For this review, take the finished solid that the model builds, in its own axes (mm). Face numbers are marked on the shaded views. Give positions to 0.01 mm unless a question says otherwise; leave off trailing zeros. Write each loop counter-clockwise with the first axis right and the second up, starting at its lowest first coordinate (ties: lowest second). Pieces come first, ordered by that corner, then holes. Notation, with made-up numbers: (-22, 46) -> (-9, 46) arc R35 cw to (-9, 84) -> close; hole circle Ø8 at (86.25, 2). An arc over 180 degrees is marked (long way). Return JSON: item names as keys, results as strings.
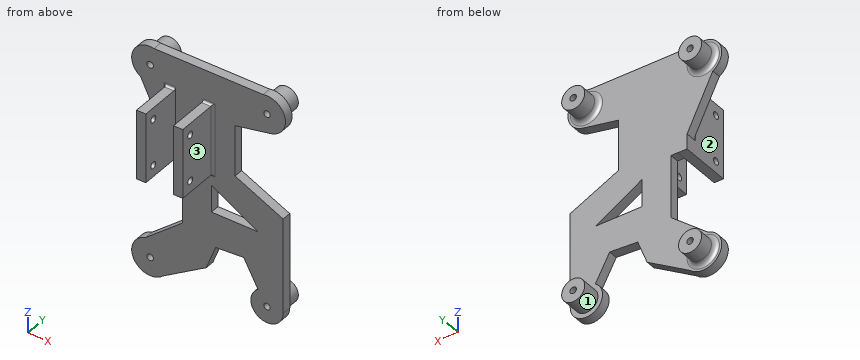
Autodesk Inventor part; units mm, degrees
ref_plane "YZ Plane" through (0, 0, 0) normal (1, 0, 0) x (0, 1, 0)
ref_plane "XZ Plane" through (0, 0, 0) normal (0, 1, 0) x (-1, 0, 0)
ref_plane "XY Plane" through (0, 0, 0) normal (0, 0, 1) x (1, 0, 0)
sketch "Sketch1" plane through (0, 0, 0) normal (0, 1, 0) x (-1, 0, 0)
  line L0 (0, 0) -> (25.3, 0) construction
  line L1 (25.3, 0) -> (25.3, -42) construction
  line L2 (25.3, -42) -> (0, -42) construction
  line L3 (0, -42) -> (0, 0) construction
  circle A0 centre (25.3, 0) radius 2.5
  circle A1 centre (0, 0) radius 2.5
  circle A2 centre (0, -42) radius 2.5
  circle A3 centre (25.3, -42) radius 2.5
  dimension "d0" = 25.3
  dimension "d1" = 42
  dimension "d2" = 5
  dimension "d3" = 5
  dimension "d4" = 5
  dimension "d5" = 5
extrude "Extrusion1" add sketch "Sketch1" along normal blind 6
sketch "Sketch2" plane through (0, 0, 0) normal (0, 1, 0) x (-1, 0, 0)
  circle A0 centre (0, 0) radius 2.5
  arc A1 (0.8438, 3.91) -> (-0.7933, -3.9205) centre (0, 0) ccw
  arc A2 (27.3626, -3.4272) -> (24.4562, 3.91) centre (25.3, 0) ccw
  circle A3 centre (25.3, -42) radius 2.5
  arc A4 (22.5627, -44.9167) -> (26.3151, -38.1309) centre (25.3, -42) ccw
  circle A5 centre (0, -42) radius 2.5
  arc A6 (-3.5, -42) -> (1.9296, -39.08) centre (0, -42) ccw
  line L0 (26.3151, -38.1309) -> (18.3, -31.5476)
  line L1 (0.8438, 3.91) -> (24.4562, 3.91)
  line L2 (6.9132, -16.448) -> (6.9132, -5.4484)
  line L3 (6.9132, -5.4484) -> (-0.7933, -3.9205)
  line L4 (18.3, -31.5476) -> (18.3, -18.0196)
  line L5 (-3.5, -42) -> (-3.5, -21.4061)
  line L6 (-3.5, -21.4061) -> (6.9132, -16.448)
  line L7 (22.5627, -44.9167) -> (13.1542, -39.1017)
  line L8 (13.1542, -39.1017) -> (11.1047, -33.8253)
  line L9 (11.1047, -33.8253) -> (5.0372, -33.4161)
  line L10 (35.6, -30.5) -> (19.8, -30.5) construction
  line L11 (19.8, -30.5) -> (19.8, -14.4) construction
  line L12 (19.8, -14.4) -> (35.6, -14.4) construction
  line L13 (35.6, -14.4) -> (35.6, -30.5) construction
  circle A7 centre (8, -39.2) radius 4.55 construction
  line L14 (-2.3049, -15.9586) -> (4, -15.9586) construction
  line L15 (4, -15.9586) -> (4, -6.2) construction
  line L16 (4, -6.2) -> (-2.3049, -6.2) construction
  line L17 (-2.3049, -6.2) -> (-2.3049, -15.9586) construction
  line L18 (5.0372, -33.4161) -> (1.9296, -39.08)
  line L19 (12.0305, -26.4894) -> (1.9134, -26.4894)
  line L20 (1.9134, -26.4894) -> (12.0305, -20.5783)
  line L21 (12.0305, -20.5783) -> (12.0305, -26.4894)
  line L22 (18.3, -18.0196) -> (20.2183, -18.0196)
  line L23 (20.2183, -18.0196) -> (27.3626, -3.4272)
  dimension "d8" = 8
  dimension "d9" = 8
  dimension "d10" = 8
  dimension "d11" = 7
  dimension "d15" = 7
  dimension "d18" = 15.8
  dimension "d19" = 11.5
  dimension "d20" = 16.1
  dimension "d21" = 2.8
  dimension "d22" = 8
  dimension "d23" = 9.1
  dimension "d24" = 6.2
  dimension "d25" = 4
  dimension "d26" = 9.7586
  dimension "d27" = 6.3049
  dimension "d28" = 5.5
extrude "Extrusion2" add sketch "Sketch2" along normal blind 2
hole "Hole1" at (-25.3, 6, 0) direction (0, -1, 0) diameter 1.4 depth 8 tip angle 118
hole "Hole2" at (-25.3, 6, -42) direction (0, -1, 0) diameter 1.4 depth 8 tip angle 118
hole "Hole3" at (0, 6, -42) direction (0, -1, 0) diameter 1.4 depth 8 tip angle 118
hole "Hole4" at (0, 6, 0) direction (0, -1, 0) diameter 1.4 depth 8 tip angle 118
sketch "Sketch3" plane through (0, 0, 0) normal (0, 1, 0) x (-1, 0, 0)
  line L0 (21.8, -18.05) -> (19.8, -18.05)
  line L1 (19.8, -18.05) -> (19.8, -3.05)
  line L2 (19.8, -3.05) -> (21.8, -3.05)
  line L3 (21.8, -3.05) -> (21.8, -18.05)
  circle A0 centre (25.3, 0) radius 0.7 construction
  circle A1 centre (25.3, -42) radius 0.7 construction
  circle A2 centre (0, -42) radius 0.7 construction
  circle A3 centre (0, 0) radius 0.7 construction
  line L4 (13.8, -18.05) -> (11.8, -18.05)
  line L5 (11.8, -18.05) -> (11.8, -3.05)
  line L6 (11.8, -3.05) -> (13.8, -3.05)
  line L7 (13.8, -3.05) -> (13.8, -18.05)
  dimension "d69" = 2
  dimension "d70" = 15
  dimension "d73" = 3.5
  dimension "d74" = 18.05
  dimension "d79" = 2
  dimension "d80" = 6
extrude "Extrusion3" add sketch "Sketch3" along normal blind 2 and the other way blind 9
fillet "Fillet1" radius 1 3 edges at (-22.8, 2, -42) (2.5, 2, 0) (-22.8, 2, 0)
sketch "Sketch4" plane through (-11.8, -9, -3.05) normal (1, 0, 0) x (0, 0, -1)
  circle A0 centre (12.5084, 2.25) radius 0.75
  circle A1 centre (2.5084, 2.25) radius 0.75
  line L0 (18.3561, 9) -> (13.398, 9)
  point P0 (-3.05, 9)
  dimension "d83" = 1.5
  dimension "d84" = 10
  dimension "d85" = 6.75
extrude "Extrusion4" cut sketch "Sketch4" against normal through all
fillet "Fillet2" radius 0.5 5 edges at (-11.8, 0, -10.55) (-21.8, 0, -8.9195) (-20.8, 0, -3.05) (-12.8, 0, -3.05) (-12.8, 0, -18.05)
properties part number "gimbal_controller_holder"
1. For pin 1 (5 mm diameter, centred on x = -18.5, y = 4, fed in from +Z); pin 2 (4 mm diameter, centred on y = -5.5, z = -13, fed in from +X); pin 3 (1 mm diameter, centred on y = 1, z = -22.5, fed in from +X), all flat-tipped, find the tip position at first contact; note any pin that passes through.
Results found:
{"pin 1": "stops at z = 3.91", "pin 2": "stops at x = -11.8", "pin 3": "stops at x = 3.5"}
2. Add section A-A, the plane z = 0. State the section outline as (x, y) points.
Results found:
{"outline": "(-29.3, 0) -> (-26, 0) -> (-26, 6) -> (-27.8, 6) -> (-27.8, 3) arc R1 cw to (-28.8, 2) -> (-29.3, 2) -> close; (-24.6, 0) -> (-0.7, 0) -> (-0.7, 6) -> (-2.5, 6) -> (-2.5, 3) arc R1 cw to (-3.5, 2) -> (-21.8, 2) arc R1 cw to (-22.8, 3) -> (-22.8, 6) -> (-24.6, 6) -> close; (0.7, 0) -> (4, 0) -> (4, 2) -> (3.5, 2) arc R1 cw to (2.5, 3) -> (2.5, 6) -> (0.7, 6) -> close"}
3. The part is to be moulded in two halves that separate along X. For the marked faces 1, 2 and 3, say which applies: +X half, -X half, draft (parallel to the pull), parting line (faces both ways), or undercut.
Results found:
{"face 1": "undercut", "face 2": "-X half", "face 3": "+X half"}
4. To check wall thickness, follow probe 1 along Z at (x, y) = (-25.3, 3.05); probe 2 along X at (y, z) = (-4, -4.5); probe 3 along X at (y, z) = (0.75, -42). State the ranges of each line that lie inside material, in increasing order.
Results found:
{"probe 1": "z = -44.5 to -42.7, -41.3 to -39.5, -2.5 to -0.7, 0.7 to 2.5", "probe 2": "x = -21.8 to -19.8, -13.8 to -11.8", "probe 3": "x = -29.3 to -26, -24.6 to -17.84, -3.5 to -0.7, 0.7 to 3.5"}
5. Add section C-C, the plane y = -2.25. State the section outline as (x, z) points.
Results found:
{"outline": "(-21.8, -18.05) -> (-19.8, -18.05) -> (-19.8, -3.05) -> (-21.8, -3.05) -> close; (-13.8, -18.05) -> (-11.8, -18.05) -> (-11.8, -3.05) -> (-13.8, -3.05) -> close"}
6. Add section B-B, the plane y = -6.75. State the section outline as (x, z) points.
Results found:
{"outline": "(-21.8, -18.05) -> (-19.8, -18.05) -> (-19.8, -16.31) -> (-21.8, -16.31) -> close; (-21.8, -14.81) -> (-19.8, -14.81) -> (-19.8, -6.31) -> (-21.8, -6.31) -> close; (-21.8, -4.81) -> (-19.8, -4.81) -> (-19.8, -3.05) -> (-21.8, -3.05) -> close; (-13.8, -18.05) -> (-11.8, -18.05) -> (-11.8, -16.31) -> (-13.8, -16.31) -> close; (-13.8, -14.81) -> (-11.8, -14.81) -> (-11.8, -6.31) -> (-13.8, -6.31) -> close; (-13.8, -4.81) -> (-11.8, -4.81) -> (-11.8, -3.05) -> (-13.8, -3.05) -> close"}
7. Add section D-D, the plane x = -8. State the section outline as (y, z) points, plus the area to 3 significant figures.
Results found:
{"outline": "(0, -33.62) -> (2, -33.62) -> (2, -26.49) -> (0, -26.49) -> close; (0, -22.93) -> (2, -22.93) -> (2, 3.91) -> (0, 3.91) -> close", "area": "67.9 mm²"}
